Input: dimensioned drawing with shaded views. Units: mm. Origin: part minimum x, y, z. A direction names the side the tool comes from. Give positions to 0.01 mm unless a question says otherwise; leave off trailing zeros. Order: outer loops, then holes, each group sorted by start corner. A loop starts at its lowest first (then second) coordinate and runs counter-clockwise, first axis right, second up. Notation, with made-up numbers: (20.5, 40) -> (26.5, 40) arc R37 cw to (26.5, 76) -> close; hole circle Ø1 at (-12, 0). An arc over 180 degrees is marked (long way). One line per question, with ' | ' between items. Start each with the question number.
(1) Ray query, L1, parallel to X at y = 310, z = 297; L2, parallel to Z at x = 509, y = 82.5; L3, parallel to Z at x = 442.5, y = 146. Return the intervals inside material, ascending.
(2) First-contact query: pin 1 Ø4 at (x, z) = (224, 409) entering from +Y; pin 2 Ø2 at (x, z) = (533.5, 176.5) entering from +Y; pin 3 Ø8 at (y, z) = (208, 449.5) entering from +X. Flat tips, straight axial feed; report the tip coordinate or a pass-through.
(3) Set-up query: the marked faces 1, 2 and 3. Return all of +Z, -Z, +X, -X, +Y, -Y with unobstructed straight access to the full face (end or side cutting, diameter ignored); none if empty.
(4) Mould query, pull axis X, two halves, no side actions, for the marked faces 4, 5, 6 and 7. Classes: +X half, -X half, draft (parallel to the pull), parting line (faces both ways), or undercut.
(5) Section B-B (x = 574.5). Return loops of the section in (y, z), then the cut area to 3 significant figures.
(6) Section C-C (z = 468.5). Return loops of the section in (x, y).
(7) Section A-A (z = 329). Return loops of the section in (x, y), then the cut area to 3 significant figures.
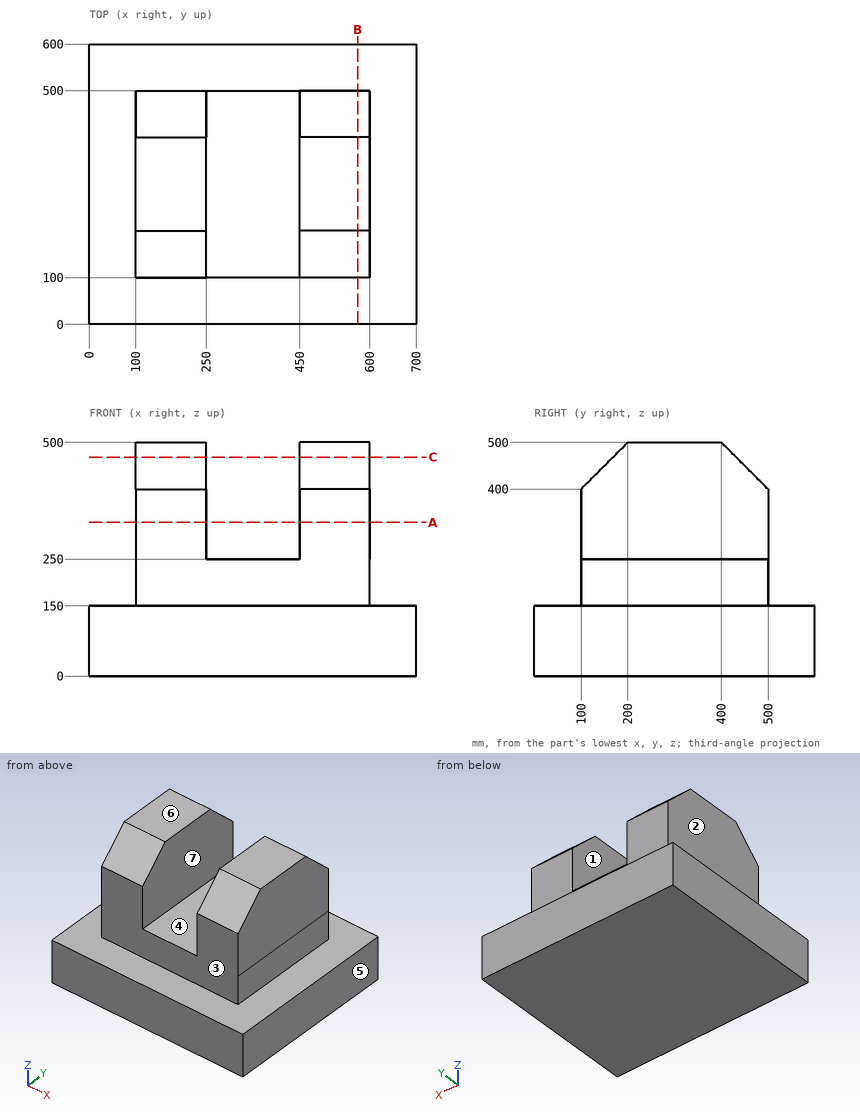
Response:
1) L1: x = 100 to 250, 450 to 600 | L2: z = 0 to 150 | L3: z = 0 to 250
2) pin 1: stops at y = 493 | pin 2: stops at y = 500 | pin 3: stops at x = 600
3) face 1: +Z, +Y, -Y | face 2: +Z, -X, +Y, -Y | face 3: +Z, +X, -X, -Y
4) face 4: undercut | face 5: +X half | face 6: draft | face 7: undercut
5) outline: (0, 0) -> (600, 0) -> (600, 150) -> (500, 150) -> (500, 400) -> (400, 500) -> (200, 500) -> (100, 400) -> (100, 150) -> (0, 150) -> close | area: 220,000 mm^2
6) outline: (100, 168.5) -> (250, 168.5) -> (250, 431.5) -> (100, 431.5) -> close; (450, 168.5) -> (600, 168.5) -> (600, 431.5) -> (450, 431.5) -> close
7) outline: (100, 100) -> (250, 100) -> (250, 500) -> (100, 500) -> close; (450, 100) -> (600, 100) -> (600, 500) -> (450, 500) -> close | area: 120,000 mm^2
